Could you check a few things on this model? Use its own coordinates, in mm. Face numbers are marked on the shaded views. A direction names the side the tool comes from. Round coordinates to 2 decimals unless told otherwise and drop trailing zeros. Write each loop counter-clockwise with the first axis right and the second up, starting at its lowest first coordinate (ties: lowest second). Pieces come first, ordered by that corner, then holes. Notation, with made-up numbers: (55, 50) - (86, 50) arc R3 ccw to (86, 54) - close; hole circle Ø8 at (-4.5, 37.5). An arc over 180 degrees is marked (long way). Put each result on its own line as item: value.
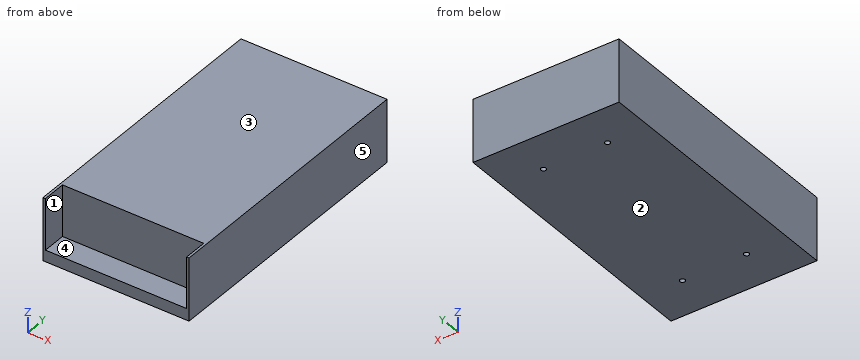
from build123d import *

# Parameters (mm, degrees)
F0_W     = 215
F0_H     = 49
F1_DEPTH = 57
F2_W     = 110.2
F2_H     = 18.5
F3_DEPTH = 40
F5_D     = 4
F5_DEPTH = 12
F5_TIP   = 1.2017212381


with BuildPart() as f1:
    # F0 (on Right) → F1 (new body, symmetric)
    with BuildSketch(Plane.YZ):
        with Locations((107.5, 24.5)):
            Rectangle(F0_W, F0_H)
    extrude(amount=F1_DEPTH, both=True)

    # F2 (on face) → F3 (cut)
    with BuildSketch(Plane.XY.offset(49)):
        with Locations((0, 9.25)):
            Rectangle(F2_W, F2_H)
    extrude(amount=-F3_DEPTH, mode=Mode.SUBTRACT)

    # F5
    with Locations(Plane(origin=(0, 0, 0), x_dir=(1, 0, 0), z_dir=(0, 0, -1))):
        with Locations((25, -32), (25, -183), (-25, -183), (-25, -32)):
            Hole(F5_D / 2, depth=F5_DEPTH)
            with Locations((0, 0, -(F5_DEPTH + F5_TIP / 2))):  # 118° drill point
                Cone(0, F5_D / 2, F5_TIP, mode=Mode.SUBTRACT)


solid = f1.part
(1) If we mould it in two halves opening along X, with no side actions, what happens to the marked faces 3, 4 and 5? For each: pulls with the +X half, pulls with the -X half, needs draft (parallel to the pull), parting line crosses it, or undercut.
Values found:
face 3: needs draft
face 4: undercut
face 5: pulls with the +X half
(2) I'm going to push flat-ended pins straight in: pin 1 (4 mm diameter, centred on x = -21.5, z = 15.5, fed in from -Y); pin 2 (10 mm diameter, centred on x = 8.5, y = 40, fed in from -Z); pin 3 (15 mm diameter, centred on x = 5, y = 7, fed in from +Z). Where does each tip first touch, or does it pass through?
Values found:
pin 1: stops at y = 18.5
pin 2: stops at z = 0
pin 3: stops at z = 9
(3) Please list where these lines run through material, in increasing order: probe 1 along X at (y, z) = (183, 9); probe 2 along X at (y, z) = (13, 42); probe 3 along Y at (x, z) = (-25, 8). Write a range as from..to.
Values found:
probe 1: x = -57..-27, -23..23, 27..57
probe 2: x = -57..-55.1, 55.1..57
probe 3: y = 0..30, 34..181, 185..215
(4) Imagine slicing it at A-A, the plane x = -38. List the corners of the cut face in (y, z) for me.
Values found:
outline: (0, 0) - (215, 0) - (215, 49) - (18.5, 49) - (18.5, 9) - (0, 9) - close
(5) For the marked faces 1 and 2, which set-ups out of +Z, -Z, +X, -X, +Y, -Y let a thin tool reach every point of the face, with its end or its side?
Values found:
face 1: +Z, -Y
face 2: -Z, +X, -X, +Y, -Y
